Geometry check sheet. Reference: the model listing, model coordinates, mm. A direction names the side the tool comes from. Coordinates: 2 decimals unless noted, no trailing zeros. Loops run counter-clockwise (first coordinate to the right, second up) from the corner with the lowest first, then second, coordinate; pieces in that order, holes last. Notation, with made-up numbers: (10.25, -9) - (28.25, -9) arc R19 cw to (28.25, 16) - close; hole circle Ø9 at (11.25, 26.25). An arc over 180 degrees is marked (long way). Write each question's results on one line, items separated by ' | '. Start each with the question number.
(1) Access from +Z, -Z, +X, -X, +Y, -Y to the whole of each face (thin tool, end or side, straight path). Record for faces 5 (the face through (124, 129, 0)), 6 (the face through (107.4, 126.18, 3.04)).
(2) Material ranges on probe 1 along X at (y, z) = (128, 2); probe 2 along X at (y, z) = (128.25, 2.65); probe 3 along X at (y, z) = (129.5, 1.7), recorded low to high.
(3) Sectioned sample at A-A (x = 136.5). Enter the section's corners in (y, z).
(4) Sectioned sample at C-C (z = 1.05). Enter the section's corners in (x, y) (3 decimals), plus the area to 3 significant figures.
(5) Go/stop test with flat-tipped pins: pin 1 Ø2 at (x, y) = (126.5, 133) entering from +Z; pin 2 Ø2 at (y, z) = (128.5, 3.5) entering from -X. Record where each tip stops, or that it passes through.
(6) Sectioned sample at B-B (y = 127). Enter the section's corners in (x, z).
(7) Sectioned sample at D-D (x = 112). Enter the section's corners in (y, z).
(8) Mould release check, pull along Y, two halves, no side actions. Record for faces 1 (the face through (134.98, 124.79, 3.04)), 2 (the face through (107.37, 129.43, 1.82)), 3 (the face through (108, 126, 3.683)), 4 (the face through (124, 122.845, 1)): pulls with the +Y half, pulls with the -Y half, needs draft (parallel to the pull), parting line crosses it, or undercut.
from build123d import *

# Parameters (mm, degrees)
EXTRUDE1_DEPTH     = 2.413
SKETCH4_R          = 3.7719
EXTRUDE3_DEPTH     = 1.27
SKETCH6_R          = 3.175
CUT_EXTRUDE1_DEPTH = 4.683


with BuildPart() as part:
    # Sketch1 → Extrude1 (new body)
    with BuildSketch(Plane.XY):
        with BuildLine():
            Line((101.766590689, 134.097427572), (144.70432984, 134.097427572))
            ThreePointArc((144.70432984, 134.097427572), (147.047960264, 128.471327572), (144.70432984, 122.845227572))
            Line((144.70432984, 122.845227572), (101.766590689, 122.845227572))
            ThreePointArc((101.766590689, 122.845227572), (99.422960264, 128.471327572), (101.766590689, 134.097427572))
        make_face()
    extrude(amount=EXTRUDE1_DEPTH)

    # Sketch4 → Extrude3 (add)
    with BuildSketch(Plane.XY.offset(2.413)):
        with Locations((135.795760264, 128.471327572)):
            Circle(SKETCH4_R)
        with Locations((110.395760264, 128.471327572)):
            Circle(SKETCH4_R)
    extrude(amount=EXTRUDE3_DEPTH)

    # Sketch6 → Cut-Extrude1 (cut, through all)
    with BuildSketch(Plane(origin=(0, 0, 0), x_dir=(-1, 0, 0), z_dir=(0, 0, -1))):
        with Locations((-135.795760264, 128.471327572)):
            Circle(SKETCH6_R)
        with Locations((-110.395760264, 128.471327572)):
            Circle(SKETCH6_R)
    extrude(amount=-CUT_EXTRUDE1_DEPTH, mode=Mode.SUBTRACT)


solid = part.part
Outcome:
1) face 5: -Z, +X, -X, +Y, -Y | face 6: +Z
2) probe 1: x = 99.44 to 107.26, 113.54 to 132.66, 138.94 to 147.03 | probe 2: x = 106.63 to 107.23, 113.56 to 114.16, 132.03 to 132.63, 138.96 to 139.56 | probe 3: x = 99.49 to 107.39, 113.4 to 132.79, 138.8 to 146.98
3) outline: (122.85, 0) - (125.38, 0) - (125.38, 3.68) - (124.77, 3.68) - (124.77, 2.41) - (122.85, 2.41) - close; (131.57, 0) - (134.1, 0) - (134.1, 2.41) - (132.18, 2.41) - (132.18, 3.68) - (131.57, 3.68) - close
4) outline: (101.767, 122.845) - (144.704, 122.845) arc R7.925 ccw to (144.704, 134.097) - (101.767, 134.097) arc R7.925 ccw to start; hole circle Ø6.35 at (110.396, 128.471); hole circle Ø6.35 at (135.796, 128.471) | area: 456 mm2
5) pin 1: stops at z = 2.41 | pin 2: stops at x = 106.62
6) outline: (99.56, 0) - (107.58, 0) - (107.58, 3.68) - (106.92, 3.68) - (106.92, 2.41) - (99.56, 2.41) - close; (113.21, 0) - (132.98, 0) - (132.98, 3.68) - (132.32, 3.68) - (132.32, 2.41) - (113.87, 2.41) - (113.87, 3.68) - (113.21, 3.68) - close; (138.61, 0) - (146.91, 0) - (146.91, 2.41) - (139.27, 2.41) - (139.27, 3.68) - (138.61, 3.68) - close
7) outline: (122.85, 0) - (125.73, 0) - (125.73, 3.68) - (125.06, 3.68) - (125.06, 2.41) - (122.85, 2.41) - close; (131.21, 0) - (134.1, 0) - (134.1, 2.41) - (131.89, 2.41) - (131.89, 3.68) - (131.21, 3.68) - close
8) face 1: parting line crosses it | face 2: undercut | face 3: needs draft | face 4: pulls with the -Y half
